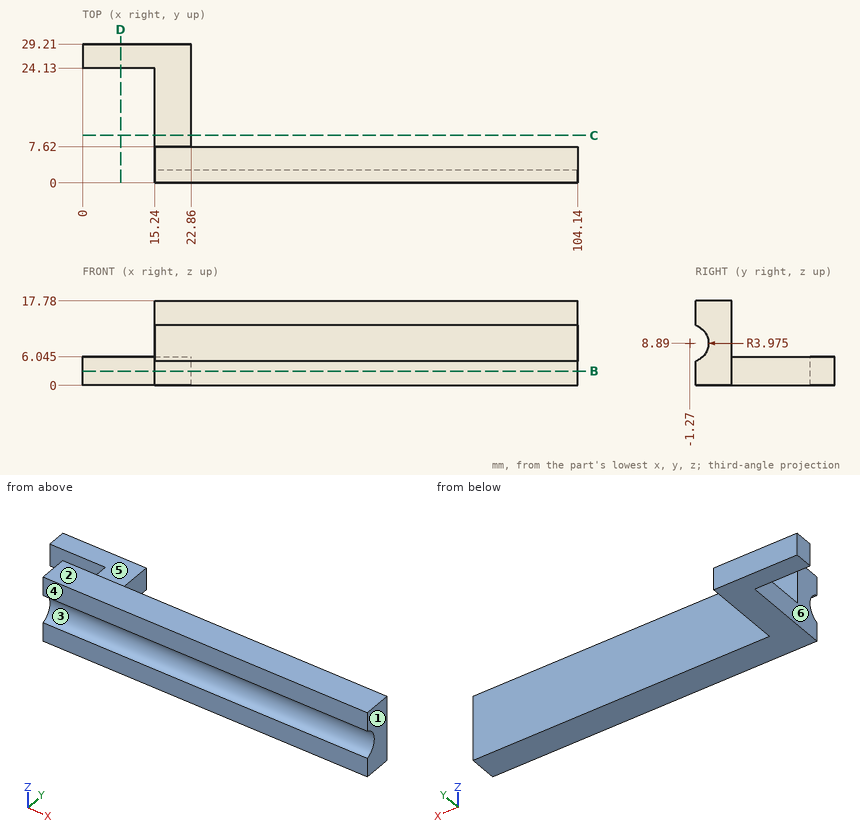
Answer from the drawing. Dimensions are ordinates in mm from the lowest x, y and z of the part. A direction names the side the tool comes from. Coordinates: 2 decimals unless noted, no trailing zeros. Write each loop counter-clockwise with the first axis right and the second up, starting at its lowest first coordinate (ties: lowest second). Pieces come first, ordered by that corner, then holes. Notation, with made-up numbers: M 87.25,-36.75 L 141.25,-36.75 A31 ccw 141.25,-3.75 Z; hole C 71,39 d5. An arc over 180 degrees is marked long. Use one line per item in the form item = value. Start each with the question number.
1. The part is cut by section D-D (x = 8). Give the vertices of the cut face in (y, z) (1 decimal).
2. The part is cut by section C-C (y = 10). Give the vertices of the cut face in (x, z) (1 decimal), plus the area to 3 significant figures.
3. A tool of negligible diameter and unlimited length cuts with its end or side. For the marked faces 4, 5 and 6, from which of +Z, -Z, +X, -X, +Y, -Y can it reach the whole face along a straight path? Write none if from no direction.
4. Each of these flat-tipped pins is pushed along its axis until it touches: P1, Ø6, axis at x = 18, z = 12.5, coming from the +Y side; P2, Ø6.5, axis at x = 4, z = 3.5, coming from the -Y side; P3, Ø1.5, axis at y = 4.5, z = 14, coming from the -X side; P4, Ø10, axis at x = 30.5, y = 19, coming from the +Z side. Where does it stop, or does it pass through?
5. The part is cut by section B-B (z = 3). Give the vertices of the cut face in (x, y).
6. The mould has two halves that part along Z. Classify the marked faces 1, 2 and 3: released by +Z, released by -Z, zero draft, split by the parting line, or undercut.
7. Straight lines are drawn through the part: probe 1 along Y at (x, z) = (21, 15); probe 2 along Y at (x, z) = (4, 3); probe 3 along X at (y, z) = (19, 1.25). For each, find the intervals that lie inside material, in ascending order. Write a range as from..to.
Evaluation:
q1.outline = M 24.1,0 L 29.2,0 L 29.2,6 L 24.1,6 Z
q2.outline = M 15.2,0 L 22.9,0 L 22.9,6 L 15.2,6 Z
q2.area = 46.1 mm^2
q3.face_4 = +Z, -Z, +X, -X, -Y
q3.face_5 = +Z, +X, -X, +Y
q3.face_6 = +Z, -Z, -X, -Y
q4.P1 = 7.62
q4.P2 = 24.13
q4.P3 = 15.24
q4.P4 = through
q5.outline = M 0,24.13 L 15.24,24.13 L 15.24,0 L 104.14,0 L 104.14,7.62 L 22.86,7.62 L 22.86,29.21 L 0,29.21 Z
q6.face_1 = zero draft
q6.face_2 = released by +Z
q6.face_3 = undercut
q7.probe_1 = 0..7.62
q7.probe_2 = 24.13..29.21
q7.probe_3 = 15.24..22.86
